Here's how the part is built. I have some questions about the finished solid (model axes, mm). A direction names the side the tool comes from. Round coordinates to 2 decimals unless told otherwise and drop trailing zeros. Order: outer loops, then holes, each group sorted by start corner. A loop starts at its lowest first (then second) coordinate and runs counter-clockwise, first axis right, second up. Notation, with made-up numbers: (4.5, 68) -> (57.5, 68) arc R20 ccw to (57.5, 86) -> close; hole circle Ø9 at (46.5, 12.25). An arc over 180 degrees is marked (long way). One line per item, written item: value.
Autodesk Inventor part; units mm, degrees
ref_plane "ANBAU_XY" through (0, 0, 0) normal (0, 0, 1) x (1, 0, 0)
ref_plane "ANBAU_YZ" through (0, 0, 0) normal (1, 0, 0) x (0, 1, 0)
ref_plane "ANBAU_ZX" through (0, 0, 0) normal (0, 1, 0) x (0, 0, 1)
sketch "Skizze_1" plane through (0, 0, 0) normal (1, 0, 0) x (0, 1, 0)
  line L0 (0, 0) -> (0, 7.6)
  line L1 (6.2894, 7.6) -> (5, 7.6)
  line L2 (5, 7.6) -> (4.594, 7.194)
  line L3 (4.594, 7.194) -> (4.594, 0.406)
  line L4 (4.594, 0.406) -> (5, 0)
  line L5 (5, 0) -> (7.5, 0)
  line L6 (7.5, 0) -> (7.5, 0.3)
  line L7 (7.5, 0.3) -> (9, 0.3)
  line L8 (9, 0.3) -> (9, 5.1)
  line L9 (9, 5.1) -> (7.45, 5.3733)
  line L10 (7.45, 5.3733) -> (6.7593, 7.271)
  arc A0 (6.7593, 7.271) -> (6.2894, 7.6) centre (6.2894, 7.1) ccw
revolve "Revolution1" add sketch "Skizze_1" angle 360 about axis through (0, 0, 0) along (0, 0, -1)
thread "Thread1"
sketch "Skizze_2" plane through (0, 0, 0) normal (0, 0, 1) x (1, 0, 0)
  line L0 (-18, 18) -> (-18, -18)
  line L1 (-18, -18) -> (18, -18)
  line L2 (18, -18) -> (18, 18)
  line L3 (18, 18) -> (-18, 18)
  arc A0 (-9.8869, -1.5) -> (-1.5, -9.8869) centre (0, 0) ccw
  line L4 (-1.5, -9.8869) -> (-1.5, -7.3485)
  arc A1 (-1.5, -7.3485) -> (1.5, -7.3485) centre (0, 0) ccw
  line L5 (1.5, -7.3485) -> (1.5, -9.8869)
  arc A2 (1.5, -9.8869) -> (9.8869, -1.5) centre (0, 0) ccw
  line L6 (9.8869, -1.5) -> (7.3485, -1.5)
  arc A3 (7.3485, -1.5) -> (7.3485, 1.5) centre (0, 0) ccw
  line L7 (7.3485, 1.5) -> (9.8869, 1.5)
  arc A4 (9.8869, 1.5) -> (1.5, 9.8869) centre (0, 0) ccw
  line L8 (1.5, 9.8869) -> (1.5, 7.3485)
  arc A5 (1.5, 7.3485) -> (-1.5, 7.3485) centre (0, 0) ccw
  line L9 (-1.5, 7.3485) -> (-1.5, 9.8869)
  arc A6 (-1.5, 9.8869) -> (-9.8869, 1.5) centre (0, 0) ccw
  line L10 (-9.8869, 1.5) -> (-7.3485, 1.5)
  arc A7 (-7.3485, 1.5) -> (-7.3485, -1.5) centre (0, 0) ccw
  line L11 (-7.3485, -1.5) -> (-9.8869, -1.5)
extrude "Extrusion1" cut sketch "Skizze_2" along normal blind 7.6
ref_plane "ANBAU_XY" through (0, 0, 0) normal (0, 0, 1) x (1, 0, 0)
ref_plane "ANBAU_YZ" through (0, 0, 0) normal (1, 0, 0) x (0, 1, 0)
ref_plane "ANBAU_ZX" through (0, 0, 0) normal (0, 1, 0) x (0, 0, 1)
properties part number "717739 GUK M10x0.75"
Q1. Which directions (+Z, -Z, +X, -X, +Y, -Y) give clear straight access to the entire face, cutting with the end or side of a thin tool? Please do faces 1 (the face through (8, -1.5, 3)), 2 (the face through (1.5, 8, 3)), 3 (the face through (1.5, -8, 3)), 4 (the face through (5.5, -5.5, 0.3)).
Answers:
face 1: +Z, -Z, +X
face 2: +Z, -Z, +Y
face 3: +Z, -Z, -Y
face 4: -Z, +X, -Y
Q2. I want a section at C-C on z = 4. Write out the boundary of the cut face in (x, y), then the cut area to 3 significant figures.
Answers:
outline: (-8.87, -1.5) arc R9 ccw to (-1.5, -8.87) -> (-1.5, -7.35) arc R7.5 ccw to (1.5, -7.35) -> (1.5, -8.87) arc R9 ccw to (8.87, -1.5) -> (7.35, -1.5) arc R7.5 ccw to (7.35, 1.5) -> (8.87, 1.5) arc R9 ccw to (1.5, 8.87) -> (1.5, 7.35) arc R7.5 ccw to (-1.5, 7.35) -> (-1.5, 8.87) arc R9 ccw to (-8.87, 1.5) -> (-7.35, 1.5) arc R7.5 ccw to (-7.35, -1.5) -> close; hole circle Ø9.19 at (0, 0)
area: 170 mm2
Q3. For P1, Ø1.2, axis at x = -8, z = 4, coming from the +Y side; P2, Ø0.5, axis at x = -8, z = 3.5, coming from the -Y side; P3, Ø0.5, axis at y = -8.5, z = 2, coming from the -X side; P4, Ø1, axis at x = -3.5, y = 1.5, coming from the -Z side (1 decimal), each with a flat end and sliding along its axis, tell me the tip position at first contact or that it passes through.
Answers:
P1: y = 5.12
P2: y = -4.58
P3: x = -3.6
P4: through
Q4. I need wall thicknesses on line 1 along X through (y, z) = (0, 3.75); line 2 along Y through (x, z) = (3.25, 6.5); line 3 along X through (y, z) = (3.75, 3). Which ranges of each line are inside material? Lowest first, please.
Answers:
line 1: -7.5 to -4.59, 4.59 to 7.5
line 2: -6.24 to -3.25, 3.25 to 6.24
line 3: -8.18 to -2.65, 2.65 to 8.18
Q5. I want a section at A-A on y = 0. Write out the boundary of the cut face in (x, z).
Answers:
outline: (-7.5, 0) -> (-5, 0) -> (-4.59, 0.41) -> (-4.59, 7.19) -> (-5, 7.6) -> (-6.29, 7.6) arc R0.5 ccw to (-6.76, 7.27) -> (-7.45, 5.37) -> (-7.5, 5.36) -> close; (4.59, 0.41) -> (5, 0) -> (7.5, 0) -> (7.5, 5.36) -> (7.45, 5.37) -> (6.76, 7.27) arc R0.5 ccw to (6.29, 7.6) -> (5, 7.6) -> (4.59, 7.19) -> close
